Geometry: final body of the model. Coordinates: model frame, mm. Round coordinates to 2 decimals unless told otherwise and drop trailing zeros. Return JSON: item names as keys, results as strings.
from build123d import *

# Parameters (mm, degrees)
SKETCH1_W           = 101.6
SKETCH1_H           = 6.35
BOSS_EXTRUDE1_DEPTH = 635
SKETCH2_R           = 6.54812
SKETCH2_R_2         = 5.0419
CUT_EXTRUDE1_DEPTH  = 6.35


with BuildPart() as part:
    # Sketch1 → Boss-Extrude1 (new body)
    with BuildSketch(Plane(origin=(0, 0, 0), x_dir=(1, 0, 0), z_dir=(0, 1, 0))):
        with Locations((50.8, 3.175)):
            Rectangle(SKETCH1_W, SKETCH1_H)
    extrude(amount=BOSS_EXTRUDE1_DEPTH)

    # Sketch2 → Cut-Extrude1 (cut)
    with BuildSketch(Plane.XY):
        with Locations((25.4, 28.575)):
            Circle(SKETCH2_R)
        with Locations((76.2, 28.575)):
            Circle(SKETCH2_R)
        with Locations((15.24, 210.312)):
            Circle(SKETCH2_R_2)
        with Locations((86.36, 210.312)):
            Circle(SKETCH2_R_2)
        with Locations((15.24, 177.292)):
            Circle(SKETCH2_R_2)
        with Locations((86.36, 177.292)):
            Circle(SKETCH2_R_2)
        with Locations((15.24, 578.612)):
            Circle(SKETCH2_R_2)
        with Locations((15.24, 545.592)):
            Circle(SKETCH2_R_2)
        with Locations((86.36, 578.612)):
            Circle(SKETCH2_R_2)
        with Locations((86.36, 545.592)):
            Circle(SKETCH2_R_2)
    extrude(amount=-CUT_EXTRUDE1_DEPTH, mode=Mode.SUBTRACT)


solid = part.part
Q1. Pull-direction query (Y, two-part tool) for faces 1 (the cylindrical face through (82.446, 30.542, -3.131)), 2 (the flat face through (50, 313, -6.35)), 3 (the cylindrical face through (17.57, 172.82, -3.13)); classes: pulls with the +Y half, pulls with the -Y half, needs draft (parallel to the pull), parting line crosses it, or undercut.
Determined:
{"face 1": "undercut", "face 2": "needs draft", "face 3": "undercut"}
Q2. Pin query (flat end, axial travel): pin 1 (1.5 mm diameter, centred on x = 58, z = -1, fed in from -Y). Return the tip coordinate at first contact, or that it passes through.
Determined:
{"pin 1": "stops at y = 0"}
Q3. Material intervals for L1, parallel to Y at x = 86.36, z = -4; L2, parallel to Y at x = 84, z = -3; L3, parallel to Y at x = 26, z = -1.25, sorted ascending.
Determined:
{"L1": "y = 0 to 172.25, 182.33 to 205.27, 215.35 to 540.55, 550.63 to 573.57, 583.65 to 635", "L2": "y = 0 to 172.84, 181.75 to 205.86, 214.77 to 541.14, 550.05 to 574.16, 583.07 to 635", "L3": "y = 0 to 22.05, 35.1 to 635"}
